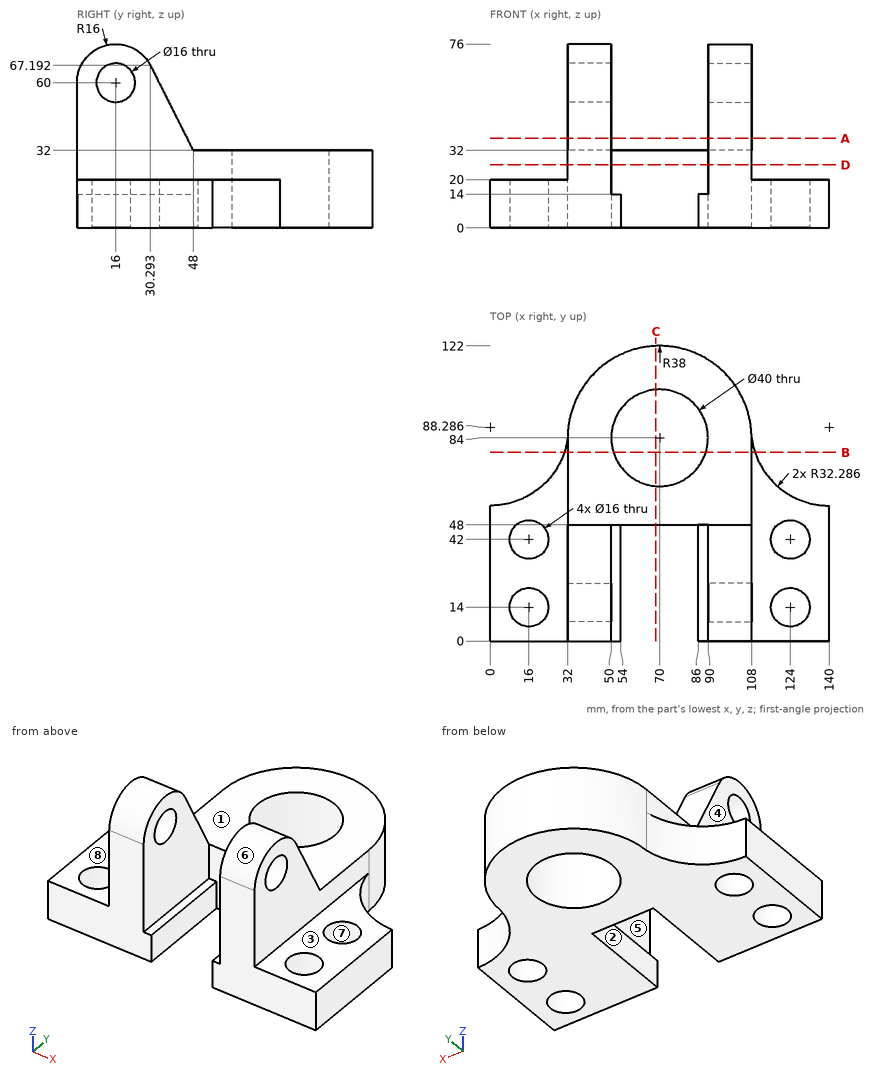
Study the drawing (mm; zero at the part's minimum x, y, z) and answer. A direction names the side the tool comes from. Give positions to 0.01 mm unless a question says otherwise; leave off trailing zeros. Write each loop counter-clockwise with the first axis right and the second up, starting at its lowest first coordinate (ties: lowest second). Pieces come first, ordered by that corner, then holes. Notation, with made-up numbers: (-29, 27.25) - (0, 27.25) arc R24 ccw to (0, 41.25) - close; hole circle Ø7 at (-1, 33.5). An arc over 180 degrees is marked (long way). Use CSV: the item, a comma, the result in double quotes. Start each with the question number.
(1) Find section C-C (x = 68.5). Give the vertices of the cut face in (y, z).
(2) Find section A-A (z = 37). Give the vertices of the cut face in (x, y).
(3) Determine the mould class of the marked faces 6, 7 and 8 for opening direction Y: +Y half, -Y half, draft (parallel to the pull), parting line (faces both ways), or undercut.
(4) Given P1, Ø4, axis at y = 76, z = 30.5, coming from the -X side; P2, Ø5, axis at y = 65, z = 19, coming from the -X side; P3, Ø4.5, axis at x = 88, y = 26.5, coming from the +Z side (1 decimal), each flat-ended and moving along its own axis, determine where each tip first touches the part or whether it passes through.
(5) Find section B-B (y = 78). Give the vertices of the cut face in (x, z).
(6) Find section D-D (z = 26). Give the vertices of the cut face in (x, y).
(7) Consider line 1 along Y through (x, z) = (124, 14) (1 decimal); line 2 along Y through (x, z) = (120.5, 16.5) (1 decimal); line 3 along Y through (x, z) = (70, 9). Determine where each line is inside the solid, lowest interval first.
(8) For the marked faces 1, 2, 3, 4 and 5, determine the directions among +Z, -Z, +X, -X, +Y, -Y from which every point of the face is accessible in a straight line to the end or side of a thin tool.
Findings below:
1,outline,"(48, 0) - (64.06, 0) - (64.06, 32) - (48, 32) - close; (103.94, 0) - (121.97, 0) - (121.97, 32) - (103.94, 32) - close"
2,outline,"(32, 0) - (50, 0) - (50, 45.48) - (32, 45.48) - close; (90, 0) - (108, 0) - (108, 45.48) - (90, 45.48) - close"
3,face 6,"parting line"
3,face 7,"undercut"
3,face 8,"draft"
4,P1,"x = 32"
4,P2,"x = 19.43"
4,P3,"z = 72.9"
5,outline,"(30.6, 0) - (50.92, 0) - (50.92, 32) - (32, 32) - (32, 20) - (30.6, 20) - close; (89.08, 0) - (109.4, 0) - (109.4, 20) - (108, 20) - (108, 32) - (89.08, 32) - close"
6,outline,"(32, 0) - (50, 0) - (50, 48) - (90, 48) - (90, 0) - (108, 0) - (108, 84) arc R38 ccw to (32, 84) - close; hole circle Ø40 at (70, 84)"
7,line 1,"0 to 6, 22 to 34, 50 to 60.2"
7,line 2,"0 to 6.8, 21.2 to 34.8, 49.2 to 62.6"
7,line 3,"48 to 64, 104 to 122"
8,face 1,"+Z, +X, -X, +Y"
8,face 2,"+Z, -Z, -Y"
8,face 3,"+Z, +X, +Y, -Y"
8,face 4,"+Z, -X, +Y, -Y"
8,face 5,"+Z, -Y"
